Build history of the part. All positions in model axes, mm. Face numbers are marked on the shaded views. A direction names the side the tool comes from. Give positions to 0.01 mm unless a question says otherwise; leave off trailing zeros. Order: outer loops, then holes, each group sorted by start corner. A loop starts at its lowest first (then second) coordinate and runs counter-clockwise, first axis right, second up. Notation, with made-up numbers: M 89.25,14 L 109.25,14 A26 cw 109.25,35 Z; hole C 65,-19.5 d3. An arc over 180 degrees is marked long. Answer as CSV lines item,"result".
from build123d import *

# Parameters (mm, degrees)
SKETCH1_W           = 125
SKETCH1_H           = 62
SKETCH1_R           = 7.5
BOSS_EXTRUDE2_DEPTH = 12
SKETCH1_3_W         = 125
SKETCH1_3_H         = 12
BOSS_EXTRUDE3_DEPTH = 62
SKETCH1_4_W         = 125
SKETCH1_4_H         = 12
BOSS_EXTRUDE4_DEPTH = 12
CUT_EXTRUDE1_REACH  = 154.686
SKETCH3_R           = 6
SKETCH4_W           = 12
SKETCH4_H           = 74
BOSS_EXTRUDE5_DEPTH = 15
SKETCH5_W           = 12
SKETCH5_H           = 62
BOSS_EXTRUDE6_DEPTH = 50
CUT_EXTRUDE2_REACH  = 130.286


with BuildPart() as part:
    # Sketch1 → Boss-Extrude2 (new body)
    with BuildSketch(Plane(origin=(0, 0, 0), x_dir=(1, 0, 0), z_dir=(0, 1, 0))):
        with Locations((62.5, 31)):
            Rectangle(SKETCH1_W, SKETCH1_H)
        with Locations(Location((110, 47, 0), (0, 0, 270))):
            Circle(SKETCH1_R, mode=Mode.SUBTRACT)
        with Locations(Location((15, 15, 0), (0, 0, 270))):
            Circle(SKETCH1_R, mode=Mode.SUBTRACT)
    extrude(amount=BOSS_EXTRUDE2_DEPTH)

    # Sketch1_3 → Boss-Extrude3 (add)
    with BuildSketch(Plane(origin=(0, 0, 0), x_dir=(1, 0, 0), z_dir=(0, 1, 0))):
        with Locations((62.5, 68)):
            Rectangle(SKETCH1_3_W, SKETCH1_3_H)
    extrude(amount=BOSS_EXTRUDE3_DEPTH)

    # Sketch1_4 → Boss-Extrude4 (add)
    with BuildSketch(Plane(origin=(0, 0, 0), x_dir=(1, 0, 0), z_dir=(0, 1, 0))):
        with Locations((62.5, 68)):
            Rectangle(SKETCH1_4_W, SKETCH1_4_H)
    extrude(amount=-BOSS_EXTRUDE4_DEPTH)

    # Sketch3 → Cut-Extrude1 (cut, up to next)
    with BuildSketch(Plane.XY.offset(-62), mode=Mode.PRIVATE) as cut_extrude1_sk1:
        with Locations((105, 42)):
            Circle(SKETCH3_R)
    cut_extrude1_tool1 = extrude(cut_extrude1_sk1.sketch, amount=-CUT_EXTRUDE1_REACH, mode=Mode.PRIVATE) & part.part
    # Sketch3 → Cut-Extrude1 (cut, up to next)
    with BuildSketch(Plane.XY.offset(-62), mode=Mode.PRIVATE) as cut_extrude1_sk2:
        with Locations((20, 32)):
            Circle(SKETCH3_R)
    cut_extrude1_tool2 = extrude(cut_extrude1_sk2.sketch, amount=-CUT_EXTRUDE1_REACH, mode=Mode.PRIVATE) & part.part
    # Sketch3 → Cut-Extrude1 (cut, up to next)
    with BuildSketch(Plane.XY.offset(-62), mode=Mode.PRIVATE) as cut_extrude1_sk3:
        with BuildLine():
            Line((115, 62), (125, 62))
            Line((125, 62), (125, 52))
            ThreePointArc((125, 52), (122.071067812, 59.071067812), (115, 62))
        make_face()
    cut_extrude1_tool3 = extrude(cut_extrude1_sk3.sketch, amount=-CUT_EXTRUDE1_REACH, mode=Mode.PRIVATE) & part.part
    # Sketch3 → Cut-Extrude1 (cut, up to next)
    with BuildSketch(Plane.XY.offset(-62), mode=Mode.PRIVATE) as cut_extrude1_sk4:
        with BuildLine():
            Line((0, 62), (0, 52))
            ThreePointArc((0, 52), (2.928932188, 59.071067812), (10, 62))
            Line((10, 62), (0, 62))
        make_face()
    cut_extrude1_tool4 = extrude(cut_extrude1_sk4.sketch, amount=-CUT_EXTRUDE1_REACH, mode=Mode.PRIVATE) & part.part
    add(cut_extrude1_tool1.solids().sort_by_distance((105, 42, -62))[0], mode=Mode.SUBTRACT)
    add(cut_extrude1_tool2.solids().sort_by_distance((20, 32, -62))[0], mode=Mode.SUBTRACT)
    add(cut_extrude1_tool3.solids().sort_by_distance((122.766321, 59.766321, -62))[0], mode=Mode.SUBTRACT)
    add(cut_extrude1_tool4.solids().sort_by_distance((2.233679, 59.766321, -62))[0], mode=Mode.SUBTRACT)

    # Sketch4 → Boss-Extrude5 (add)
    with BuildSketch(Plane(origin=(0, 0, -74), x_dir=(-1, 0, 0), z_dir=(0, 0, -1))):
        with Locations((-78.5, 25)):
            Rectangle(SKETCH4_W, SKETCH4_H)
        with Locations((-46.5, 25)):
            Rectangle(SKETCH4_W, SKETCH4_H)
    extrude(amount=BOSS_EXTRUDE5_DEPTH)

    # Sketch5 → Boss-Extrude6 (add)
    with BuildSketch(Plane(origin=(0, 12, 0), x_dir=(1, 0, 0), z_dir=(0, 1, 0))):
        with Locations((62.5, 31)):
            Rectangle(SKETCH5_W, SKETCH5_H)
    extrude(amount=BOSS_EXTRUDE6_DEPTH)

    # Sketch6 → Cut-Extrude2 (cut, up to next)
    with BuildSketch(Plane(origin=(68.5, 0, 0), x_dir=(0, 0, -1), z_dir=(1, 0, 0)), mode=Mode.PRIVATE) as cut_extrude2_sk1:
        Polygon((0, 12), (62, 47.79571669), (62, 62), (0, 62), align=None)
    cut_extrude2_tool1 = extrude(cut_extrude2_sk1.sketch, amount=-CUT_EXTRUDE2_REACH, mode=Mode.PRIVATE) & part.part
    add(cut_extrude2_tool1.solids().sort_by_distance((68.5, 44.285835, -25.238872))[0], mode=Mode.SUBTRACT)


solid = part.part
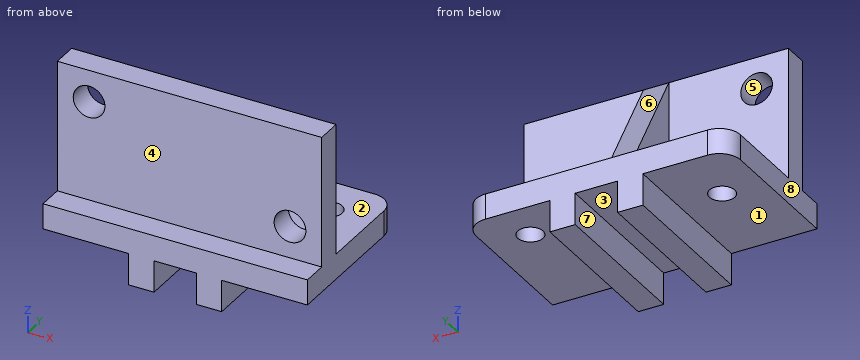
Item 1: Drop flat-ended pins along their axis: pin 1 (20 mm diameter, centred on x = 107.5, y = 7, fed in from -Z); pin 2 (18 mm diameter, centred on y = 31, z = -36.5, fed in from -X); pin 3 (4 mm diameter, centred on x = 92, z = -58, fed in from -Y). Give the stop position or say it passes through.
Geometry says:
pin 1,"stops at z = -74"
pin 2,"stops at x = 56.5"
pin 3,"stops at y = 0"
Item 2: Band-saw the part on D-D (y = 30). Give the cut face in (x, z), and give its area (3 significant figures).
Geometry says:
outline,"M 0,-74 L 14.34,-74 L 14.34,-62 L 0,-62 Z; M 25.66,-74 L 40.5,-74 L 40.5,-89 L 52.5,-89 L 52.5,-74 L 72.5,-74 L 72.5,-89 L 84.5,-89 L 84.5,-74 L 125,-74 L 125,-62 L 68.5,-62 L 68.5,-31.18 L 56.5,-31.18 L 56.5,-62 L 25.66,-62 Z"
area,"2,090 mm2"
Item 3: Band-saw the part on B-B (y = 8.5). Give the cut face in (x, z), and give its area (3 significant figures).
Geometry says:
outline,"M 0,-74 L 40.5,-74 L 40.5,-89 L 52.5,-89 L 52.5,-74 L 72.5,-74 L 72.5,-89 L 84.5,-89 L 84.5,-74 L 125,-74 L 125,0 L 0,0 Z; hole C 15,-15 d15; hole C 110,-47 d15"
area,"9,260 mm2"
Item 4: Probe line 1 along Y through (x, z) = (105, -71.25); line 2 along X through (y, z) = (8, -47); line 3 along X through (y, z) = (11, -83). List the from-to ranges inside material, lowest first. Write a range as from..to.
Geometry says:
line 1,"y = -12..36, 48..62"
line 2,"x = 0..102.5, 117.5..125"
line 3,"x = 40.5..52.5, 72.5..84.5"
Item 5: 3-axis set-ups, long thin cutter, end or side, ignore diameter. For the marked faces 1, 2, 3 and 4: which of +Z, -Z, +X, -X, +Y, -Y reach the whole face in a straight line?
Geometry says:
face 1,"-Z, -X, +Y, -Y"
face 2,"+Z, +Y"
face 3,"-Z, +Y, -Y"
face 4,"+Z, +X, -X, -Y"
Item 6: Pull direction X, two halves, no side cores. Call the marked faces 5, 6, 7 and 8: released by +X, released by -X, zero draft, split by the parting line, or undercut.
Geometry says:
face 5,"undercut"
face 6,"zero draft"
face 7,"undercut"
face 8,"released by -X"
Item 7: Band-saw the part on C-C (x = 59.5). Give the cut face in (y, z), and give its area (3 significant figures).
Geometry says:
outline,"M -12,-74 L 62,-74 L 62,-62 L 47.8,-62 L 12,0 L 0,0 L 0,-62 L -12,-62 Z"
area,"2,740 mm2"
Item 8: Band-saw the part on A-A (z = -77). Give the cut face in (x, y), and give its area (3 significant figures).
Geometry says:
outline,"M 40.5,-12 L 52.5,-12 L 52.5,62 L 40.5,62 Z; M 72.5,-12 L 84.5,-12 L 84.5,62 L 72.5,62 Z"
area,"1,780 mm2"
